```python
from build123d import *

# Parameters (mm, degrees)
SKETCH1_R            = 50.5
SKETCH1_R_2          = 45
SKETCH1_R_3          = 40
BOSS_EXTRUDE1_DEPTH  = 40
FILLET1_R            = 5
FILLET2_R            = 5
CUT_EXTRUDE1_START   = -0.5
SKETCH2_R            = 41.5
SKETCH2_R_2          = 40
CUT_EXTRUDE1_DEPTH   = 0.5
SKETCH3_R            = 1
BOSS_EXTRUDE2_DEPTH  = 5
SKETCH4_R            = 12
BOSS_EXTRUDE3_DEPTH  = 7.5
CUT_EXTRUDE2_DEPTH   = 5
SKETCH6_R            = 6
CUT_EXTRUDE3_DEPTH   = 79.259184829
BOSS_EXTRUDE10_START = -12.5
BOSS_EXTRUDE10_DEPTH = 12.5
CIRPATTERN2_START    = 27
CIRPATTERN2_DEPTH    = 12.5
SKETCH8_R            = 45.5
CUT_EXTRUDE4_DEPTH   = 82.85658196


# Read off the part's stored shape, not the designer's step: Boss-Extrude10, CirPattern2, Cut-Revolve1
with BuildPart() as part:
    # Sketch1 → Boss-Extrude1 (new body)
    # profile 1 of 2: a face of its own
    with BuildSketch(Plane(origin=(0, 0, 0), x_dir=(1, 0, 0), z_dir=(0, 1, 0))):
        with Locations(Location((0, 0, 0), (0, 0, 270))):
            Circle(SKETCH1_R)
        Circle(SKETCH1_R_2, mode=Mode.SUBTRACT)
    # profile 2 of 2: a face of its own
    with BuildSketch(Plane(origin=(0, 0, 0), x_dir=(1, 0, 0), z_dir=(0, 1, 0))):
        Circle(SKETCH1_R_2)
        with Locations(Location((0, 0, 0), (0, 0, 270))):
            Circle(SKETCH1_R_3, mode=Mode.SUBTRACT)
    extrude(amount=BOSS_EXTRUDE1_DEPTH)

    # Fillet1
    fillet1_edges = [part.edges().sort_by_distance(p)[0] for p in [
        (0, 40, -50.5),
    ]]
    fillet(fillet1_edges, radius=FILLET1_R)

    # Fillet2
    fillet2_edges = [part.edges().sort_by_distance(p)[0] for p in [
        (0, 0, -50.5),
    ]]
    fillet(fillet2_edges, radius=FILLET2_R)

    # Sketch2 → Cut-Extrude1 (cut)
    with BuildSketch(Plane(origin=(0, 40, 0), x_dir=(1, 0, 0), z_dir=(0, 1, 0)).offset(CUT_EXTRUDE1_START)):
        with Locations(Location((0, 0, 0), (0, 0, 270))):
            Circle(SKETCH2_R)
        with Locations(Location((0, 0, 0), (0, 0, 270))):
            Circle(SKETCH2_R_2, mode=Mode.SUBTRACT)
    extrude(amount=CUT_EXTRUDE1_DEPTH, mode=Mode.SUBTRACT)


with BuildPart() as body_2:
    # Sketch3 → Boss-Extrude2 (new body)
    with BuildSketch(Plane(origin=(0, 39.5, 0), x_dir=(1, 0, 0), z_dir=(0, 1, 0))):
        with Locations(Location((0, 0, 0), (0, 0, 270))):
            Circle(SKETCH3_R)
    extrude(amount=-BOSS_EXTRUDE2_DEPTH)

    # Sketch4 → Boss-Extrude3 (add)
    with BuildSketch(Plane.XZ.offset(-34.5)):
        with Locations(Location((0, 0, 0), (0, 0, 270))):
            Circle(SKETCH4_R)
    extrude(amount=BOSS_EXTRUDE3_DEPTH)

    # Sketch5 → Cut-Extrude2 (cut)
    with BuildSketch(Plane.XZ.offset(-27)):
        Polygon((1.172923904, 10.937287119), (-8.885506541, 6.484425457), (-10.058430445, -4.452861662), (-1.172923904, -10.937287119), (8.885506541, -6.484425457), (10.058430445, 4.452861662), align=None)
    extrude(amount=-CUT_EXTRUDE2_DEPTH, mode=Mode.SUBTRACT)

    # Sketch6 → Cut-Extrude3 (cut, through all)
    with BuildSketch(Plane.XZ.offset(-32)):
        with Locations(Location((0, 0, 0), (0, 0, 270))):
            Circle(SKETCH6_R)
    extrude(amount=-CUT_EXTRUDE3_DEPTH, mode=Mode.SUBTRACT)

    # Boss-Extrude10 outline → Boss-Extrude10 (add)
    with BuildSketch(Plane(origin=(0, 39.5, 0), x_dir=(1, 0, 0), z_dir=(0, 1, 0)).offset(BOSS_EXTRUDE10_START)):
        with BuildLine():
            ThreePointArc((-9.907874683, -6.770082663), (-10.682049717, -5.467523557), (-11.285904868, -4.077787551))
            ThreePointArc((-11.285904868, -4.077787551), (-11.291897259, -4.637537864), (-11.663342081, -5.056327867))
            Line((-11.663342081, -5.056327867), (-14.441281094, -6.530254709))
            ThreePointArc((-14.441281094, -6.530254709), (-15.188724822, -6.754494743), (-15.965085937, -6.675633223))
            Line((-15.965085937, -6.675633223), (-39.993984407, 0.693693915))
            ThreePointArc((-39.993984407, 0.693693915), (-39.913717484, -2.625863016), (-39.558397626, -5.927324632))
            ThreePointArc((-39.558397626, -5.927324632), (-38.549233859, -3.209595167), (-35.711897206, -2.614628217))
            Line((-35.711897206, -2.614628217), (-16.968675274, -8.362912276))
            ThreePointArc((-16.968675274, -8.362912276), (-16.496554918, -8.752791347), (-16.438401548, -9.362316987))
            Line((-16.438401548, -9.362316987), (-22.186706389, -28.105606681))
            ThreePointArc((-22.186706389, -28.105606681), (-24.270105502, -30.121529322), (-27.086328062, -29.433498469))
            ThreePointArc((-27.086328062, -29.433498469), (-25.333453103, -30.955066692), (-23.495271849, -32.372398749))
            Line((-23.495271849, -32.372398749), (-22.678682838, -32.949618279))
            Line((-22.678682838, -32.949618279), (-21.84791965, -33.506244298))
            Line((-21.84791965, -33.506244298), (-14.474389556, -9.463641401))
            ThreePointArc((-14.474389556, -9.463641401), (-14.104425603, -8.776547206), (-13.499682622, -8.283335601))
            Line((-13.499682622, -8.283335601), (-10.652684086, -6.77276696))
            ThreePointArc((-10.652684086, -6.77276696), (-10.280610826, -6.679459968), (-9.907874683, -6.770082663))
        make_face()
    extrude(amount=BOSS_EXTRUDE10_DEPTH)

    # CirPattern2 outline → CirPattern2 (add)
    with BuildSketch(Plane(origin=(0, 0, 0), x_dir=(1, 0, 0), z_dir=(0, 1, 0)).offset(CIRPATTERN2_START)):
        with BuildLine():
            ThreePointArc((-9.500432888, 7.330878183), (-8.500858804, 8.469675294), (-7.365742824, 9.473427714))
            ThreePointArc((-7.365742824, 9.473427714), (-7.899948758, 9.306154457), (-8.413024481, 9.530006248))
            Line((-8.413024481, 9.530006248), (-10.673242573, 11.716514805))
            ThreePointArc((-10.673242573, 11.716514805), (-11.117480333, 12.358082052), (-11.282387348, 13.120814899))
            Line((-11.282387348, 13.120814899), (-11.699078736, 38.250902692))
            ThreePointArc((-11.699078736, 38.250902692), (-14.831361144, 37.148764806), (-17.861437852, 35.790627793))
            ThreePointArc((-17.861437852, 35.790627793), (-14.964874781, 35.670680608), (-13.522242341, 33.156067994))
            Line((-13.522242341, 33.156067994), (-13.197211247, 13.553887176))
            ThreePointArc((-13.197211247, 13.553887176), (-13.422115065, 12.984394777), (-13.983838017, 12.740733854))
            Line((-13.983838017, 12.740733854), (-33.586089702, 12.415701585))
            ThreePointArc((-33.586089702, 12.415701585), (-36.147151798, 13.774177532), (-36.363056203, 16.665177575))
            ThreePointArc((-36.363056203, 16.665177575), (-37.268485425, 14.527903984), (-38.048419067, 12.341710032))
            Line((-38.048419067, 12.341710032), (-38.345047581, 11.386717087))
            Line((-38.345047581, 11.386717087), (-38.61771044, 10.424607444))
            Line((-38.61771044, 10.424607444), (-13.473290178, 10.841536484))
            ThreePointArc((-13.473290178, 10.841536484), (-12.705499618, 10.70200364), (-12.049551649, 10.279269655))
            Line((-12.049551649, 10.279269655), (-9.733144569, 8.038404527))
            ThreePointArc((-9.733144569, 8.038404527), (-9.529427386, 7.713375274), (-9.500432888, 7.330878183))
        make_face()
        with BuildLine():
            ThreePointArc((4.03628425, 11.300814548), (5.428230042, 10.702070763), (6.73362545, 9.932687868))
            ThreePointArc((6.73362545, 9.932687868), (6.409460418, 10.389057624), (6.463807004, 10.946195641))
            Line((6.463807004, 10.946195641), (7.844854414, 13.771459088))
            ThreePointArc((7.844854414, 13.771459088), (8.317744107, 14.392209487), (8.992187082, 14.784742791))
            Line((8.992187082, 14.784742791), (32.763556111, 22.946664049))
            ThreePointArc((32.763556111, 22.946664049), (30.747432198, 25.585062307), (28.519421945, 28.047149087))
            ThreePointArc((28.519421945, 28.047149087), (29.300432607, 25.255288185), (27.354691835, 23.106205171))
            Line((27.354691835, 23.106205171), (8.812350166, 16.739675231))
            ThreePointArc((8.812350166, 16.739675231), (8.201231607, 16.777588643), (7.795914361, 17.23652355))
            Line((7.795914361, 17.23652355), (1.429361404, 35.778932255))
            ThreePointArc((1.429361404, 35.778932255), (1.929937095, 38.634439204), (4.612723394, 39.733144639))
            ThreePointArc((4.612723394, 39.733144639), (2.300262401, 39.933805139), (-0.019944352, 39.999995028))
            Line((-0.019944352, 39.999995028), (-1.019859867, 39.986996459))
            Line((-1.019859867, 39.986996459), (-2.01913797, 39.949006018))
            Line((-2.01913797, 39.949006018), (6.147438285, 16.164079439))
            ThreePointArc((6.147438285, 16.164079439), (6.251994995, 15.390749203), (6.052650154, 14.636273627))
            Line((6.052650154, 14.636273627), (4.637269925, 11.740774173))
            ThreePointArc((4.637269925, 11.740774173), (4.391100809, 11.446588055), (4.03628425, 11.300814548))
        make_face()
        with BuildLine():
            ThreePointArc((11.994993743, -0.346590692), (11.855689469, -1.855431813), (11.52735222, -3.334689012))
            ThreePointArc((11.52735222, -3.334689012), (11.861213145, -2.885363735), (12.407876906, -2.764885294))
            Line((12.407876906, -2.764885294), (15.521629237, -3.205285014))
            ThreePointArc((15.521629237, -3.205285014), (16.258128901, -3.463207416), (16.839864598, -3.98334134))
            Line((16.839864598, -3.98334134), (31.948070005, -24.069084381))
            ThreePointArc((31.948070005, -24.069084381), (33.834319309, -21.336326696), (35.487409954, -18.45653637))
            ThreePointArc((35.487409954, -18.45653637), (33.073538017, -20.062054114), (30.428371647, -18.875647848))
            Line((30.428371647, -18.875647848), (18.643543171, -3.208198923))
            ThreePointArc((18.643543171, -3.208198923), (18.490754948, -2.615274747), (18.801978065, -2.087976452))
            Line((18.801978065, -2.087976452), (34.469483632, 9.69689463))
            ThreePointArc((34.469483632, 9.69689463), (37.339918519, 10.103219032), (39.213876041, 7.891256292))
            ThreePointArc((39.213876041, 7.891256292), (38.690125771, 10.152544892), (38.036092779, 12.379646445))
            Line((38.036092779, 12.379646445), (37.714739519, 13.326605833))
            Line((37.714739519, 13.326605833), (37.369814547, 14.265236092))
            Line((37.369814547, 14.265236092), (17.272615982, -0.851585994))
            ThreePointArc((17.272615982, -0.851585994), (16.569445022, -1.18999752), (15.790295166, -1.233555084))
            Line((15.790295166, -1.233555084), (12.599134998, -0.782207034))
            ThreePointArc((12.599134998, -0.782207034), (12.243276933, -0.638994801), (11.994993743, -0.346590692))
        make_face()
        with BuildLine():
            ThreePointArc((3.377029578, -11.515019376), (1.89898901, -11.848790687), (0.390670022, -11.99363902))
            ThreePointArc((0.390670022, -11.99363902), (0.921172454, -12.172310482), (1.204682652, -12.654988728))
            Line((1.204682652, -12.654988728), (1.748040016, -15.75243417))
            ThreePointArc((1.748040016, -15.75243417), (1.730332147, -16.53258938), (1.415421606, -17.246583128))
            Line((1.415421606, -17.246583128), (-13.018562973, -37.822176274))
            ThreePointArc((-13.018562973, -37.822176274), (-9.836672879, -38.7716374), (-6.586996421, -39.453915879))
            ThreePointArc((-6.586996421, -39.453915879), (-8.859861984, -37.654319512), (-8.548923935, -34.7719971))
            Line((-8.548923935, -34.7719971), (2.709993184, -18.722451208))
            ThreePointArc((2.709993184, -18.722451208), (3.226683428, -18.393917326), (3.824347139, -18.526963966))
            Line((3.824347139, -18.526963966), (19.873951055, -29.785921788))
            ThreePointArc((19.873951055, -29.785921788), (21.147401687, -32.390306446), (19.62278483, -34.856080037))
            ThreePointArc((19.62278483, -34.856080037), (21.611550355, -33.659187323), (23.527542489, -32.348952756))
            Line((23.527542489, -32.348952756), (24.328850767, -31.7507011))
            Line((24.328850767, -31.7507011), (25.114953513, -31.132605256))
            Line((25.114953513, -31.132605256), (4.527625467, -16.690388528))
            ThreePointArc((4.527625467, -16.690388528), (3.988485204, -16.126208116), (3.706288951, -15.398652596))
            Line((3.706288951, -15.398652596), (3.149423732, -12.224204706))
            ThreePointArc((3.149423732, -12.224204706), (3.17566047, -11.841508561), (3.377029578, -11.515019376))
        make_face()
    extrude(amount=CIRPATTERN2_DEPTH)

    # Cut-Revolve1 outline → Cut-Revolve1 (revolve, cut)
    with BuildSketch(Plane.XY):
        with BuildLine():
            Line((12, 39.5), (12, 34.5))
            add(Edge.make_bspline(
                [(12, 34.5), (18.404764838, 39.5), (40, 39.5)],
                knots=[0, 0, 0, 1, 1, 1], degree=2))
            Line((40, 39.5), (12, 39.5))
        make_face()
    revolve(axis=Axis((0, 0, 0), (0, 1, 0)), mode=Mode.SUBTRACT)


with BuildPart() as cut_extrude4_tool:
    # Sketch8 → Cut-Extrude4 (new, through all)
    with BuildSketch(Plane(origin=(0, 40, 0), x_dir=(1, 0, 0), z_dir=(0, 1, 0))):
        with Locations(Location((0, 0, 0), (0, 0, 270))):
            Circle(SKETCH8_R)
    extrude(amount=-CUT_EXTRUDE4_DEPTH)


with BuildPart() as part_1:
    add(part.part)

    # Cut-Extrude4: cut by cut_extrude4_tool
    add(cut_extrude4_tool.part, mode=Mode.SUBTRACT)


with BuildPart() as body_2_1:
    add(body_2.part)

    # Cut-Extrude4: cut by cut_extrude4_tool
    add(cut_extrude4_tool.part, mode=Mode.SUBTRACT)


solid = part_1.part
```
Check sheet for the modelled part. Datum: model origin and axes. Units: mm. Round coordinates to 2 decimals unless told otherwise and drop trailing zeros. Order: outer loops, then holes, each group sorted by start corner. A loop starts at its lowest first (then second) coordinate and runs counter-clockwise, first axis right, second up. Notation, with made-up numbers: (78, -19) -> (130, -19) arc R20 cw to (130, -9) -> close; hole circle Ø8 at (-12.5, 69). An arc over 180 degrees is marked (long way). One line per item, written item: value. Start each with the question number.
Q1. Thickness scan on line 1 (X direction, y = 8.5, z = 0); line 2 (X direction, y = 29.5, z = -5.5); line 3 (Z direction, x = 25, y = 22.5). Record the ranges inside material, lowest first.
Q2. Cross-section at C-C (y = 31). Record the boundary of the cut face in (x, z).
Q3. Gauge pin test, flat ends, axial feed: pin 1 Ø12 at (x, y) = (-8, 21) entering from -Z; pin 2 Ø8 at (x, y) = (28, 8) entering from +Z; pin 3 Ø5 at (x, y) = (4, 14.5) entering from +Z. Record the tip position at first contact, or that the pin passes through.
Q4. Cross-section at B-B (x = 0). Record the boundary of the cut face in (y, z), and give its area (3 significant figures).
Q5. Cross-section at A-A (z = 0). Record the boundary of the cut face in (x, y), and give its area (3 significant figures).
Q6. Mould release check, pull along X, two halves, no side actions. Record for faces 1 (the face through (-30.728, 19.79, -40.075)), 2 (the face through (-27.686, 20.28, -36.107)): pulls with the +X half, pulls with the -X half, needs draft (parallel to the pull), parting line crosses it, or undercut.
Completed:
1. line 1: x = -50.5 to -45.5, 45.5 to 50.5
1. line 2: x = -50.2 to -45.17, 45.17 to 50.2
1. line 3: z = -43.88 to -38.02, 38.02 to 43.88
2. outline: circle Ø101 at (0, 0); hole circle Ø91 at (0, 0)
3. pin 1: stops at z = -50.46
3. pin 2: stops at z = 44.43
3. pin 3: stops at z = 50.48
4. outline: (0, -45.5) arc R5 ccw to (5, -50.5) -> (35, -50.5) arc R5 ccw to (40, -45.5) -> close; (0, 45.5) -> (40, 45.5) arc R5 ccw to (35, 50.5) -> (5, 50.5) arc R5 ccw to start
4. area: 379 mm²
5. outline: (-50.5, 5) arc R5 ccw to (-45.5, 0) -> (-45.5, 40) arc R5 ccw to (-50.5, 35) -> close; (45.5, 0) arc R5 ccw to (50.5, 5) -> (50.5, 35) arc R5 ccw to (45.5, 40) -> close
5. area: 379 mm²
6. face 1: parting line crosses it
6. face 2: undercut
